Design review of the part built by this model. Coordinates are the model's own, in mm. Give positions to 0.01 mm unless a question says otherwise; leave off trailing zeros. Write each loop counter-clockwise with the first axis right and the second up, starting at its lowest first coordinate (ties: lowest second). Pieces come first, ordered by that corner, then holes. Notation, with made-up numbers: (-37, 13) -> (-28, 13) arc R24 ccw to (-28, 52) -> close; hole circle Ø11 at (-19.5, 87). An arc over 180 degrees is marked (long way). Put each result on its own line as item: value. Start each with the question number.
Autodesk Inventor part; units mm, degrees
ref_plane "Work Plane1" through (-29.7469, 0, 0) normal (0, -0.866, -0.5) x (1, 0, 0)
ref_plane "YZ Plane" through (0, 0, 0) normal (1, 0, 0) x (0, 1, 0)
ref_plane "XZ Plane" through (0, 0, 0) normal (0, 1, 0) x (-1, 0, 0)
sketch "Эскиз1" plane through (0, 0, 0) normal (1, 0, 0) x (0, 1, 0)
  line L0 (-13.8564, 0) -> (-6.9282, 12)
  line L1 (-6.9282, 12) -> (6.9282, 12)
  line L2 (6.9282, 12) -> (13.8564, 0)
  line L3 (13.8564, 0) -> (6.9282, -12)
  line L4 (6.9282, -12) -> (-6.9282, -12)
  line L5 (-6.9282, -12) -> (-13.8564, 0)
  point P0 (0, 0)
  point P1 (0, 0)
  dimension "d0" = 27.7128
extrude "Базовый элемент" add sketch "Эскиз1" along normal blind 8
sketch "Эскиз2" plane through (0, 0, 0) normal (0, 0, 1) x (1, 0, 0)
  line L0 (0, 6.9282) -> (0, 13.8564)
  line L1 (0, 13.8564) -> (8, 13.8564)
  line L2 (8, 6.9282) -> (8, 13.8564)
  line L3 (-1.6, 0) -> (9.6, 0)
  line L4 (1.5048, 13.8564) -> (0, 11.25)
  line L5 (6.4952, 13.8564) -> (8, 11.25)
  dimension "d3" = 30
  dimension "d4" = 30
  dimension "d5" = 22.5
  dimension "d6" = 22.5
revolve "Фаска1" cut sketch "Эскиз2" angle 360 about axis through (-10, 0, 0) along (1, 0, 0)
sketch "Эскиз3" plane through (8, 0, 0) normal (1, 0, 0) x (0, 0, -1)
  arc A0 (-0.625, -1.0825) -> (0.625, -1.0825) centre (0, 0) ccw
hole "Резьба" at (8, 0, 0) direction (-1, 0, 0) diameter 13.835 end through all
chamfer "Фаска2" distance 1.0825 angle 30 1 edges at (8, 0, 6.9175) measured on face at (8, 9.6801, -1.1754)
chamfer "Фаска3" distance 1.0825 angle 30 1 edges at (0, 0, 6.9175) measured on face at (0, 9.6801, -1.1754)
ref_plane "Work Plane1" through (-29.7469, 0, 0) normal (0, -0.866, -0.5) x (1, 0, 0)
equation "\"d0\" = 1.1547 * SW"
equation "\"d1\" = KOH"
equation "\"d3\" = ANG1"
equation "\"d4\" = ANG2"
equation "\"d5\" = SW0"
equation "\"d6\" = SW01"
equation "\"d8\" = -0.5 * GD1 + 0.5 * NND"
equation "\"d40\" = -0.5 * GD1 + 0.5 * NND"
equation "\"d10\" = -0.5 * GD1 + 0.5 * NND"
equation "\"d41\" = -0.5 * GD1 + 0.5 * NND"
equation "\"ANG1\" = 30deg"
equation "\"ANG2\" = 30deg"
equation "\"NND\" = 16"
equation "\"KOH\" = 8"
equation "\"SW\" = 24"
equation "\"SW0\" = 22.5"
equation "\"SW01\" = SW0"
equation "\"GUL\" = 0.541266 * PTC"
equation "\"LADI\" = 0"
equation "\"TOA\" = 30deg"
equation "\"FAWI\" = 30deg"
equation "\"PTC\" = 2"
equation "\"THREADDIA\" = 16"
equation "\"E0\" = 1.155 * SW"
equation "\"GAL\" = 0.541266 * PTC"
properties part number "M16-6H ГОСТ 4035-2014" material "Сталь, мягкая"
Q1. Take a section at A-A on y = 0. Give the boundary of the cut face in (x, z), then the cut area to 3 significant figures.
Q2. To check wall thickness, follow probe 1 along Z at (x, y) = (5.75, 0); probe 2 along Z at (x, y) = (5.5, 5); probe 3 along Y at (x, z) = (1, -2). State the ranges of each line that lie inside material, in increasing order. Write a range as from..to.
Q3. For pin 1 (11 mm diameter, centred on y = 0, z = 0, fed in from +X); pin 2 (2 mm diameter, centred on x = 2, z = 8, fed in from -Y), all flat-tipped, find the tip position at first contact; note any pin that passes through.
Q4. Mouldability with a two-part tool opening along Y and no side actions: class faces 1 (the face through (4, 0, 12)), 2 (the face through (3.95, -0.3, 6.91)), 3 (the face through (3.95, -10.344, -6.084)) as +Y half, -Y half, draft (parallel to the pull), parting line (faces both ways), or undercut.
Q5. Take a section at B-B on x = 4.25. Give the boundary of the cut face in (y, z) (1 decimal).
Result:
1. outline: (0, -11.25) -> (0.43, -12) -> (7.57, -12) -> (8, -11.25) -> (8, -8) -> (7.38, -6.92) -> (0.62, -6.92) -> (0, -8) -> close; (0, 8) -> (0.62, 6.92) -> (7.38, 6.92) -> (8, 8) -> (8, 11.25) -> (7.57, 12) -> (0.43, 12) -> (0, 11.25) -> close
1. area: 79.3 mm^2
2. probe 1: z = -12..-6.92, 6.92..12
2. probe 2: z = -12..-4.78, 4.78..12
2. probe 3: y = -12.7..-6.62, 6.62..12.7
3. pin 1: passes through
3. pin 2: stops at y = -9.81
4. face 1: draft
4. face 2: undercut
4. face 3: -Y half
5. outline: (-13.9, 0) -> (-6.9, -12) -> (6.9, -12) -> (13.9, 0) -> (6.9, 12) -> (-6.9, 12) -> close; hole circle Ø13.8 at (0, 0)
